Autodesk Inventor part; units mm, degrees
ref_plane "YZ Plane" through (0, 0, 0) normal (1, 0, 0) x (0, 1, 0)
ref_plane "XZ Plane" through (0, 0, 0) normal (0, 1, 0) x (-1, 0, 0)
ref_plane "XY Plane" through (0, 0, 0) normal (0, 0, 1) x (1, 0, 0)
sketch "Sketch1" plane through (0, 0, 0) normal (0, 1, 0) x (-1, 0, 0)
  point P0 (0, 0)
sketch "Sketch2" plane through (0, 0, 0) normal (0, 1, 0) x (-1, 0, 0)
  line L0 (80, -80) -> (-80, -80)
  line L1 (-80, -80) -> (-80, 80)
  line L2 (-80, 80) -> (80, 80)
  line L3 (80, 80) -> (80, -80)
  line L4 (80, -80) -> (-80, 80) construction
  line L5 (-80, -80) -> (80, 80) construction
  point P0 (0, 0)
  dimension "d0" = 160
  dimension "d1" = 160
extrude "Extrusion1" add sketch "Sketch2" along normal blind 10
chamfer "Chamfer1" distance 2 angle 45 8 edges at (80, 10, 0) (0, 10, 80) (80, 5, 80) (80, 5, -80) (-80, 10, 0) (-80, 5, 80) (-80, 5, -80) (0, 10, -80)
sketch "Sketch3" plane through (0, 10, 0) normal (0, 1, 0) x (1, 0, 0)
  point P0 (0, 0)
  point P1 (0, 60)
  point P2 (-51.9615, -30)
  point P3 (51.9615, -30)
  dimension "d8" = 60
  dimension "d11" = 360
hole "Hole1" at (0, 10, -60) at (-51.9615, 10, 30) at (51.9615, 10, 30) direction (0, -1, 0) diameter 8 end through all
sketch "Sketch4" plane through (0, 10, 0) normal (0, 1, 0) x (1, 0, 0)
  circle A0 centre (0, 60) radius 4
  point P0 (0, 0)
  point P1 (-9, 60)
  point P2 (9, 60)
  dimension "d20" = 18
  dimension "d21" = 9
hole "Hole2" at (-9, 10, -60) at (9, 10, -60) direction (0, -1, 0) diameter 4 end through all
pattern_circular "Circular Pattern1" count 3 over 360 about axis through (0, -10, 0) along (0, 1, 0) of "Hole2"
sketch "Sketch5" plane through (0, 10, 0) normal (0, 1, 0) x (1, 0, 0)
  point P0 (0, 0)
  point P1 (0, 35)
  dimension "d32" = 35
hole "Hole3" at (0, 10, -35) direction (0, -1, 0) diameter 4 end through all
pattern_circular "Circular Pattern2" count 6 over 360 about axis through (0, -10, 0) along (0, 1, 0) of "Hole3"
properties part number "De_Go" material "Wood (Oak)"
Here's how the part is built. I have some questions about the finished solid (model axes, mm). Give positions to 0.01 mm unless a question says otherwise; leave off trailing zeros. Loops run counter-clockwise (first coordinate to the right, second up) from the corner with the lowest first, then second, coordinate; pieces in that order, holes last. Notation, with made-up numbers: M 74,4 L 91,4 A10 ccw 91,16 Z; hole C 48.25,52 d1. An arc over 180 degrees is marked long. Put each result on its own line as item: value. Start each with the question number.
(1) I want a section at B-B on z = -60. Please give me the cut outline in (x, y), then the cut area to 3 significant figures.
(2) I want a section at C-C on z = -35. Please give me the cut outline in (x, y).
(3) Will this pin go through, and if not, where does the flat tip stop? pin 1 Ø7 at (x, z) = (0, -60) entering from +Y.
(4) If we mould it in two halves opening along Z, with no side actions, what happens to faces 1 (the cylindrical face through (-55.927, 4.93, 29.479)), 2 (the flat face through (1, 0, 1)), 3 (the flat face through (-1, 4, -80))? For each: +Z half, -Z half, draft (parallel to the pull), parting line (faces both ways), or undercut.
(5) I need wall thicknesses on line 1 along X through (y, z) = (1.75, -17.5); line 2 along X through (y, z) = (3.5, -60); line 3 along X through (y, z) = (5.5, 30). Which ranges of each line are inside material? Lowest first, please. Write a range as [from, to].
(6) I want a section at A-A on x = -9. Please give me the cut outline in (y, z), then the cut area to 3 significant figures.
Answer block:
1. outline: M -80,0 L -11,0 L -11,10 L -78,10 L -80,8 Z; M -7,0 L -4,0 L -4,10 L -7,10 Z; M 4,0 L 7,0 L 7,10 L 4,10 Z; M 11,0 L 80,0 L 80,8 L 78,10 L 11,10 Z
1. area: 1,440 mm^2
2. outline: M -80,0 L -2,0 L -2,10 L -78,10 L -80,8 Z; M 2,0 L 80,0 L 80,8 L 78,10 L 2,10 Z
3. pin 1: through
4. face 1: undercut
4. face 2: draft
4. face 3: -Z half
5. line 1: [-80, -32.31], [-28.31, 28.31], [32.31, 80]
5. line 2: [-80, -11], [-7, -4], [4, 7], [11, 80]
5. line 3: [-80, -55.96], [-47.96, 47.96], [55.96, 80]
6. outline: M 0,-80 L 8,-80 L 10,-78 L 10,-62 L 0,-62 Z; M 0,-58 L 10,-58 L 10,78 L 8,80 L 0,80 Z
6. area: 1,560 mm^2
